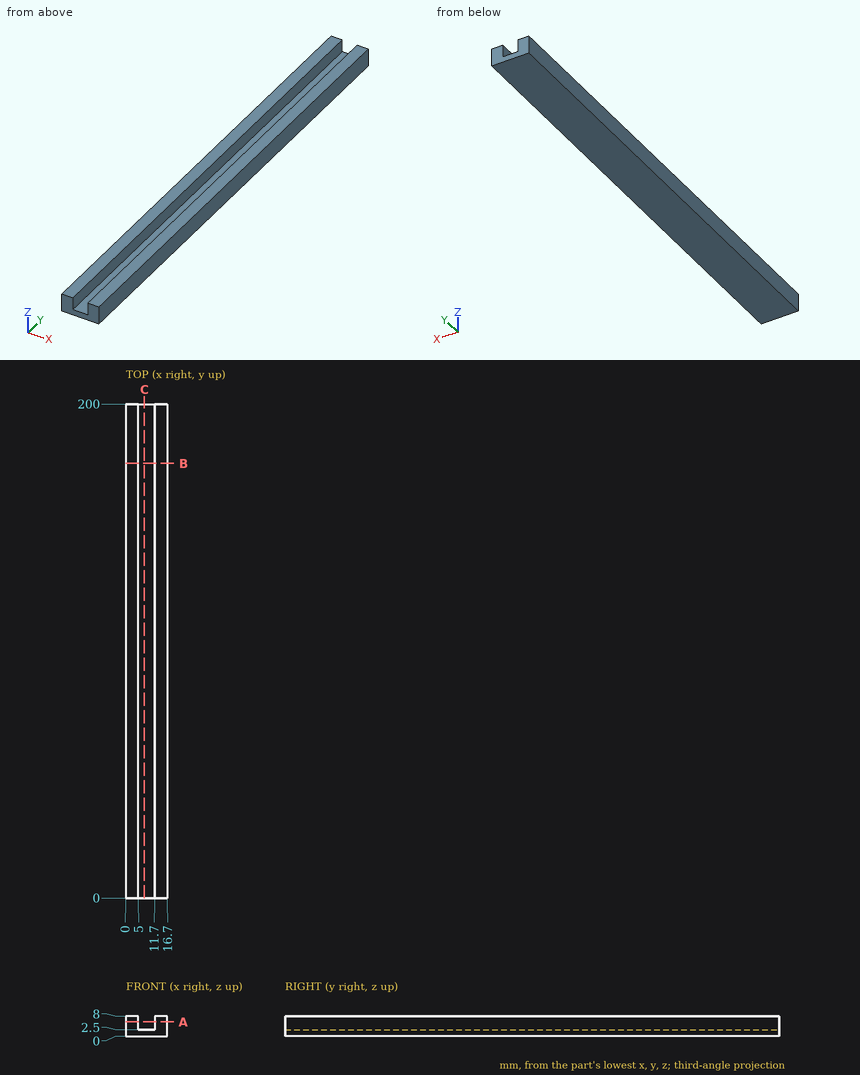
Geometry check sheet. Reference: drawing and pictorial views, mm from the part's lowest x, y, z. Give positions to 0.01 mm unless a question says otherwise; leave off trailing zeros. Loops run counter-clockwise (first coordinate to the right, second up) from the corner with the lowest first, then second, coordinate; pieces in that order, holes last.
1. Thickness scan on line 1 (X direction, y = 149, z = 3.5); line 2 (Z direction, x = 9.5, y = 127.5). Record the ranges inside material, lowest first.
2. Section check C-C, the plane x = 7.5. Enter the section's corners in (y, z), then the cut area to 3 significant figures.
3. Go/stop test with a flat-tipped pin: pin 1 Ø3 at (y, z) = (110, 4.5) entering from -X. Record where the tip stops, or that it passes through.
4. Section check A-A, the plane z = 5.75. Enter the section's corners in (x, y).
5. Section check B-B, the plane y = 176. Enter the section's corners in (x, z).
Geometry says:
1. line 1: x = 0 to 5, 11.7 to 16.7
1. line 2: z = 0 to 2.5
2. outline: (0, 0) - (200, 0) - (200, 2.5) - (0, 2.5) - close
2. area: 500 mm2
3. pin 1: stops at x = 0
4. outline: (0, 0) - (5, 0) - (5, 200) - (0, 200) - close; (11.7, 0) - (16.7, 0) - (16.7, 200) - (11.7, 200) - close
5. outline: (0, 0) - (16.7, 0) - (16.7, 8) - (11.7, 8) - (11.7, 2.5) - (5, 2.5) - (5, 8) - (0, 8) - close
